Can you work these out from the model? Positions are in its coordinate system, mm. A direction names the side the tool comes from. Give positions to 0.01 mm unless a question says otherwise; leave off trailing zeros. Order: outer loops, then holes, each group sorted by start corner. A loop starts at its lowest first (then second) coordinate and runs counter-clockwise, first axis right, second up. Notation, with made-up numbers: (43, 40) - (85, 40) arc R30 ccw to (85, 76) - close; hole circle Ø8 at (44, -14). An arc over 180 degrees is marked (long way). Write each question's results on one line, items separated by ' | '. Start each with the question number.
Solid Edge part; units mm, degrees
sketch "Sketch1" plane through (0, 0, 0) normal (0, -1, 0) x (1, 0, 0)
  line L0 (-92.067, 25.1901) -> (-52.067, 25.1901)
  line L1 (-52.067, 25.1901) -> (-52.067, 65.1901)
  line L2 (-52.067, 65.1901) -> (-92.067, 65.1901)
  line L3 (-92.067, 65.1901) -> (-92.067, 25.1901)
  line L4 (-82.067, 35.1901) -> (-62.067, 35.1901)
  line L5 (-62.067, 35.1901) -> (-62.067, 55.1901)
  line L6 (-62.067, 55.1901) -> (-82.067, 55.1901)
  line L7 (-82.067, 55.1901) -> (-82.067, 35.1901)
  dimension "D1" = 82.067
  dimension "D2" = 82.067
  dimension "D3" = 52.067
  dimension "D4" = 52.067
extrude "Protrusion1" add sketch "Sketch1" along normal blind 150
sketch "Sketch2" plane through (-52.067, -75, 45.1901) normal (1, 0, 0) x (0, 1, 0)
  circle A0 centre (-96.7389, 0) radius 5
  line L0 (-75, 20) -> (-106.7389, 7.6815)
  line L1 (-106.7389, 7.6815) -> (-106.7389, -7.6815)
  line L2 (-106.7389, -7.6815) -> (-75, -20)
  line L3 (-75, -20) -> (-75, 20)
  dimension "D1" = 106.7389
  dimension "D2" = 96.7389
extrude "ExtrudedProtrusion_2" add sketch "Sketch2" against normal blind 10
mirror "Mirror1" about plane through (-68.067, -90.8694, 45.1901) normal (1, 0, 0) of "ExtrudedProtrusion_2"
Q1. Will these pins go through, and if not, where does the flat tip stop? P1, Ø16, axis at y = -166.5, z = 49, coming from the -X side; P2, Ø9, axis at x = -89, z = 47, coming from the -Y side; P3, Ø4, axis at x = -77, z = 41.5, coming from the +Y side.
Q2. Thinking about a two-plate mould opening in X: for faces 1 (the flat face through (-88, -150, 45)), 2 (the flat face through (-74.067, -163, 45)), 3 (the flat face through (-52.067, -90, 45)), which applies, released by +X, released by -X, zero draft, split by the parting line, or undercut?
Q3. If we section it at C-C (y = -164): Please give me the cut outline in (x, z).
Q4. If I drill on probe 1 along Z at (x, y) = (-81, -60); probe 2 along X at (y, z) = (-8, 53); probe 3 along X at (y, z) = (-165, 51.5), over which ranges is the centre line in solid material (lowest first)? Write a range as from..to.
Q5. If we section it at B-B (y = -81): Please give me the cut outline in (x, z), plus the area to 3 significant figures.
Q6. Which directions (+Z, -Z, +X, -X, +Y, -Y) give clear straight access to the entire face, cutting with the end or side of a thin tool? Please do faces 4 (the flat face through (-79, -181.739, 45)), 5 (the flat face through (-79.137, -165.647, 31.263)), 6 (the flat face through (-72, -74, 35.19)), 7 (the flat face through (-84.067, -163, 45)), 8 (the flat face through (-68, -150, 60)).
Q7. If we section it at A-A (x = -72.5): Please give me the cut outline in (y, z).
Findings below:
1) P1: stops at x = -84.07 | P2: stops at y = -150 | P3: stops at y = -150
2) face 1: zero draft | face 2: undercut | face 3: released by +X
3) outline: (-84.07, 30.62) - (-74.07, 30.62) - (-74.07, 59.76) - (-84.07, 59.76) - close; (-62.07, 30.62) - (-52.07, 30.62) - (-52.07, 59.76) - (-62.07, 59.76) - close
4) probe 1: z = 25.19..35.19, 55.19..65.19 | probe 2: x = -92.07..-82.07, -62.07..-52.07 | probe 3: x = -84.07..-74.07, -62.07..-52.07
5) outline: (-92.07, 25.19) - (-52.07, 25.19) - (-52.07, 65.19) - (-92.07, 65.19) - close; hole (-82.07, 35.19) - (-62.07, 35.19) - (-62.07, 55.19) - (-82.07, 55.19) - close | area: 1,200 mm2
6) face 4: +Z, -Z, +X, -X, -Y | face 5: -Z, +X, -X, -Y | face 6: +Y | face 7: +Z, -Z, -X, -Y | face 8: +Z, -Z, -Y
7) outline: (-150, 25.19) - (0, 25.19) - (0, 35.19) - (-150, 35.19) - close; (-150, 55.19) - (0, 55.19) - (0, 65.19) - (-150, 65.19) - close
